```python
from build123d import *

# Parameters (mm, degrees)
BOX010_W           = 2
BOX010_H           = 33.5
BOX010_DEPTH       = 2
BOX011_W           = 46.1
BOX011_H           = 2
BOX011_DEPTH       = 2
BOX012_W           = 2
BOX012_H           = 33
BOX012_DEPTH       = 2
FILLET_R           = 1.99
FILLET001_R        = 1.2
FILLET002_R        = 0.99
BOX013_W           = 3
BOX013_H           = 8
BOX013_DEPTH       = 2
CHAMFER_1_ANGLE    = 50
CHAMFER_1_SIZE     = 0.499
CHAMFER_2_ANGLE    = 50
CHAMFER_2_SIZE     = 0.499
CHAMFER001_1_ANGLE = 40
CHAMFER001_1_SIZE  = 0.5955
CHAMFER001_2_ANGLE = 40
CHAMFER001_2_SIZE  = 0.5955


with BuildPart() as part:
    # Box010 → Box010 (join)
    with BuildSketch(Plane(origin=(23, -32, 2.5), x_dir=(1, 0, 0), z_dir=(0, 0, 1))):
        with Locations((1, 16.75)):
            Rectangle(BOX010_W, BOX010_H)
    extrude(amount=BOX010_DEPTH)

    # Box011 → Box011 (join)
    with BuildSketch(Plane(origin=(-23.1, -0.5, 2.5), x_dir=(1, 0, 0), z_dir=(0, 0, 1))):
        with Locations((23.05, 1)):
            Rectangle(BOX011_W, BOX011_H)
    extrude(amount=BOX011_DEPTH)

    # Box012 → Box012 (join)
    with BuildSketch(Plane(origin=(-25.1, -0.5, 2.5), x_dir=(1, 0, 0), z_dir=(0, 0, 1))):
        with Locations((1, 16.5)):
            Rectangle(BOX012_W, BOX012_H)
    extrude(amount=BOX012_DEPTH)

    # Fillet
    fillet_edges = [part.edges().sort_by_distance(p)[0] for p in [
        (-25.1, -0.5, 3.5),
        (25, 1.5, 3.5),
    ]]
    fillet(fillet_edges, radius=FILLET_R)

    # Fillet001
    fillet001_edges = [part.edges().sort_by_distance(p)[0] for p in [
        (23, -0.5, 3.5),
        (-23.1, 1.5, 3.5),
    ]]
    fillet(fillet001_edges, radius=FILLET001_R)

    # Fillet002
    fillet002_edges = [part.edges().sort_by_distance(p)[0] for p in [
        (24.417142, 0.917142, 4.5),
        (25, -16.245, 4.5),
        (0.55, 1.5, 4.5),
        (-22.748528, 1.851472, 4.5),
        (-23.1, 17.6, 4.5),
        (25, -16.245, 2.5),
        (24.417142, 0.917142, 2.5),
        (0.55, 1.5, 2.5),
        (-0.65, -0.5, 2.5),
        (22.648528, -0.851472, 2.5),
        (23, -16.85, 2.5),
        (-24.517142, 0.082858, 2.5),
        (-25.1, 16.995, 2.5),
        (-23.1, 17.6, 2.5),
        (-22.748528, 1.851472, 2.5),
        (23, -16.85, 4.5),
        (22.648528, -0.851472, 4.5),
        (-0.65, -0.5, 4.5),
        (-24.517142, 0.082858, 4.5),
        (-25.1, 16.995, 4.5),
        (-23.105, -0.5, 4.5),
    ]]
    fillet(fillet002_edges, radius=FILLET002_R)

    # Box013 → Box013 (join)
    with BuildSketch(Plane(origin=(22.5, -15, 2.5), x_dir=(1, 0, 0), z_dir=(0, 0, 1))):
        with Locations((1.5, 4)):
            Rectangle(BOX013_W, BOX013_H)
    extrude(amount=BOX013_DEPTH)

    # Chamfer 1
    chamfer_1_edges = [part.edges().sort_by_distance(p)[0] for p in [
        (22.5, -15, 3.5),
    ]]
    chamfer_1_side = part.faces().sort_by_distance((22.889504, -15, 3.5))[0]
    chamfer(chamfer_1_edges, length=CHAMFER_1_SIZE, angle=CHAMFER_1_ANGLE, reference=chamfer_1_side)

    # Chamfer 2
    chamfer_2_edges = [part.edges().sort_by_distance(p)[0] for p in [
        (25.5, -15, 3.5),
    ]]
    chamfer_2_side = part.faces().sort_by_distance((25.110496, -15, 3.5))[0]
    chamfer(chamfer_2_edges, length=CHAMFER_2_SIZE, angle=CHAMFER_2_ANGLE, reference=chamfer_2_side)

    # Chamfer001 1
    chamfer001_1_edges = [part.edges().sort_by_distance(p)[0] for p in [
        (25.5, -7, 3.5),
    ]]
    chamfer001_1_side = part.faces().sort_by_distance((25.5, -10.702657, 3.5))[0]
    chamfer(chamfer001_1_edges, length=CHAMFER001_1_SIZE, angle=CHAMFER001_1_ANGLE, reference=chamfer001_1_side)

    # Chamfer001 2
    chamfer001_2_edges = [part.edges().sort_by_distance(p)[0] for p in [
        (22.5, -7, 3.5),
    ]]
    chamfer001_2_side = part.faces().sort_by_distance((22.5, -10.702657, 3.5))[0]
    chamfer(chamfer001_2_edges, length=CHAMFER001_2_SIZE, angle=CHAMFER001_2_ANGLE, reference=chamfer001_2_side)


with BuildPart() as part_1:
    # Body001 placement: moved
    add(part.part.moved(Location((0, -0.55, 0))))


solid = part_1.part
```
Input: part model. Units: mm. Frame: model coordinates. A direction names the side the tool comes from. Give positions to 0.01 mm unless a question says otherwise; leave off trailing zeros. Write each loop counter-clockwise with the first axis right and the second up, starting at its lowest first coordinate (ties: lowest second). Pieces come first, ordered by that corner, then holes. Notation, with made-up numbers: (-14, 70) - (32, 70) arc R16 cw to (32, 101) - close; hole circle Ø9 at (30.5, 1.5). An arc over 180 degrees is marked (long way). Write item = value, one per line. Start each with the question number.
1. First-contact query: pin 1 Ø0.8 at (x, z) = (23.5, 3) entering from +Y. Flat tip, straight axial feed; report the tip coordinate or a pass-through.
2. Section query C-C, the plane z = 4. Output: boundary loops of the cut face in (x, y), then the cut area to 3 significant figures.
3. Ray query, L1, parallel to Y at x = 16, z = 3.7; L2, parallel to X at y = 12, z = 3.6; L3, parallel to X at y = -27.5, z = 3.35. Return the intervals inside material, ascending.
4. Access query for faces 1 (the flat face through (22.5, -12, 3)), 2 (the flat face through (24, -32.55, 3)). Directions: +Z, -Z, +X, -X, +Y, -Y. A direction counts if a zero-diameter tool reaches every point of the face in a straight line with its end or side. Return the directions, or none.
Check sheet entries:
q1.pin_1 = 0.92
q2.outline = (-24.97, 0.94) arc R1.86 ccw to (-23.11, -0.92) - (21.8, -0.92) arc R1.33 cw to (23.13, -2.25) - (23.13, -7.55) - (23, -7.55) - (22.5, -8.15) - (22.5, -14.96) - (23, -15.55) - (23.13, -15.55) - (23.13, -32.55) - (24.87, -32.55) - (24.87, -15.55) - (25, -15.55) - (25.5, -14.96) - (25.5, -8.15) - (25, -7.55) - (24.87, -7.55) - (24.87, -1.04) arc R1.86 ccw to (23.01, 0.82) - (-21.9, 0.82) arc R1.33 cw to (-23.23, 2.15) - (-23.23, 31.95) - (-24.97, 31.95) - close
q2.area = 205 mm2
q3.L1 = -1.03 to 0.93
q3.L2 = -25.1 to -23.1
q3.L3 = 23.01 to 24.99
q4.face_1 = +Z, -Z, -X, -Y
q4.face_2 = +Z, -Z, +X, -X, -Y
